Source: CAD feature listing. Evaluate the final solid. Frame: model axes, mm. Face numbers are marked on the shaded views. A direction names the side the tool comes from. Round coordinates to 2 decimals unless told otherwise and drop trailing zeros. Write each loop counter-clockwise with the first axis right and the second up, starting at its lowest first coordinate (ties: lowest second). Pieces come first, ordered by that corner, then holes. Notation, with made-up numbers: M 27,0 L 72,0 A24 ccw 72,33 Z; hole C -10.75,87 d7. An arc over 180 degrees is marked long. Use a Markdown table: item, result.
```python
from build123d import *

# Parameters (mm, degrees)
SKETCH1_R             = 6
BOSS_EXTRUDE1_DEPTH   = 106
SKETCH2_W             = 13.926547721
SKETCH2_H             = 4.090447759
CUT_EXTRUDE1_DEPTH    = 10
SKETCH3_R             = 1.5
CUT_EXTRUDE2_DEPTH    = 10
CHAMFER1_SIZE         = 0.5
CHAMFER1_SIZE2        = 0.866025404
CHAMFER1_PART_2_SIZE  = 0.5
CHAMFER1_PART_2_SIZE2 = 0.866025404


with BuildPart() as part:
    # Sketch1 → Boss-Extrude1 (new body)
    with BuildSketch(Plane(origin=(0, 0, 0), x_dir=(1, 0, 0), z_dir=(0, 1, 0))):
        Circle(SKETCH1_R)
    extrude(amount=BOSS_EXTRUDE1_DEPTH)

    # Sketch2 → Cut-Extrude1 (cut)
    with BuildSketch(Plane(origin=(0, 106, 0), x_dir=(1, 0, 0), z_dir=(0, 1, 0))):
        with Locations((0.543038745, 6.545223879)):
            Rectangle(SKETCH2_W, SKETCH2_H)
    extrude(amount=-CUT_EXTRUDE1_DEPTH, mode=Mode.SUBTRACT)

    # Sketch3 → Cut-Extrude2 (cut, symmetric)
    with BuildSketch(Plane(origin=(0, 0, 0), x_dir=(0, 0, -1), z_dir=(1, 0, 0))):
        with Locations((0, 5)):
            Circle(SKETCH3_R)
    extrude(amount=CUT_EXTRUDE2_DEPTH, both=True, mode=Mode.SUBTRACT)

    # Chamfer1
    chamfer1_edges = [part.edges().sort_by_distance(p)[0] for p in [
        (-6, 0, 0),
    ]]
    chamfer1_side = [part.faces().sort_by_distance(p)[0] for p in [
        (0, 0, 0),
    ]]
    chamfer(chamfer1_edges, length=CHAMFER1_SIZE, length2=CHAMFER1_SIZE2, reference=chamfer1_side[0])

    # Chamfer1 part 2
    chamfer1_part_2_edges = [part.edges().sort_by_distance(p)[0] for p in [
        (-2.468626967, 106, 5.468626967),
    ]]
    chamfer1_part_2_side = [part.faces().sort_by_distance(p)[0] for p in [
        (-6, 53, 0),
    ]]
    chamfer(chamfer1_part_2_edges, length=CHAMFER1_PART_2_SIZE, length2=CHAMFER1_PART_2_SIZE2, reference=chamfer1_part_2_side[0])


solid = part.part
```
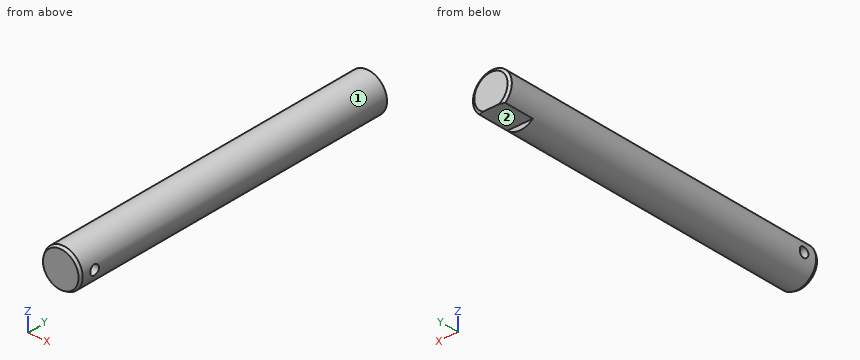
Q1. Section D-D on y = 5. Return loops of the section in (x, z).
Results are:
| item | result |
|---|---|
| outline | M -5.81,-1.5 A6 ccw 5.81,-1.5 Z; M -5.81,1.5 L 5.81,1.5 A6 ccw Z |
Q2. Line query: L1, parallel to Y at x = -2.25, z = 0; L2, parallel to Y at x = -3, z = -1.25; L3, parallel to X at y = 65.5, z = -0.5. Output: solid intervals per line, ascending.
Results are:
| item | result |
|---|---|
| L1 | 0 to 3.5, 6.5 to 106 |
| L2 | 0 to 4.17, 5.83 to 106 |
| L3 | -5.98 to 5.98 |
Q3. Section B-B on x = 0. Return loops of the section in (y, z).
Results are:
| item | result |
|---|---|
| outline | M 0,-5.5 L 0.87,-6 L 96,-6 L 96,-4.5 L 106,-4.5 L 106,5.13 L 105.5,6 L 0.87,6 L 0,5.5 Z; hole C 5,0 d3 |
Q4. Section A-A on z = 0. Return loops of the section in (x, y).
Results are:
| item | result |
|---|---|
| outline | M -6,0.87 L -5.5,0 L 5.5,0 L 6,0.87 L 6,3.5 L -6,3.5 Z; M -6,6.5 L 6,6.5 L 6,105.5 L 5.13,106 L -5.13,106 L -6,105.5 Z |
Q5. Section C-C on y = 75.5. Return loops of the section in (x, z), plus the area to 3 significant figures.
Results are:
| item | result |
|---|---|
| outline | C 0,0 d12 |
| area | 113 mm^2 |
Q6. First-contact query: pin 1 Ø6.5 at (x, y) = (1.5, 102.5) entering from -Z; pin 2 Ø3 at (y, z) = (75, -2) entering from -X; pin 3 Ø0.5 at (x, z) = (1.5, -5) entering from +Y. Flat tips, straight axial feed; report the tip coordinate or a pass-through.
Results are:
| item | result |
|---|---|
| pin 1 | z = -4.5 |
| pin 2 | x = -5.98 |
| pin 3 | y = 96 |
Q7. Reachability of the marked faces 1 and 2 from +Z, -Z, +X, -X, +Y, -Y: full face, straight path, thin tool, end or side. Return the list, or none.
Results are:
| item | result |
|---|---|
| face 1 | +Y, -Y |
| face 2 | -Z, +X, -X, +Y |
